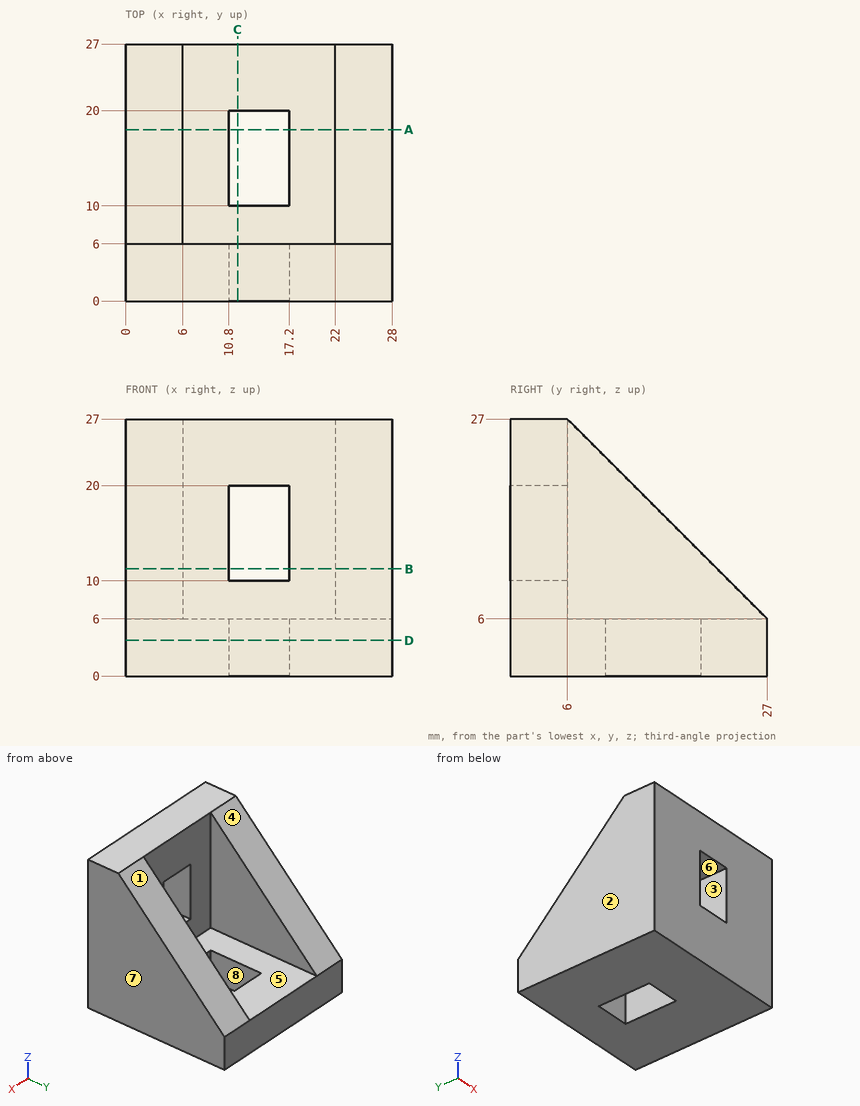
Design review of the part shown in the three views and the two pictorial views. Dimensions are in mm from the part's minimum x, y and z. A direction names the side the tool comes from. Round coordinates to 2 decimals unless told otherwise and drop trailing zeros. Write each loop counter-clockwise with the first axis right and the second up, starting at its lowest first coordinate (ties: lowest second). Pieces come first, ordered by that corner, then holes. Notation, with made-up numbers: (89.25, -20) - (122.25, -20) arc R33 ccw to (122.25, 8) - close; hole circle Ø5 at (-17, 0). An arc over 180 degrees is marked (long way). Write item = value, one per line. Start each with the question number.
1. Consider section D-D on z = 3.75. State the section outline as (x, y) points.
2. For pin 1 Ø3 at (y, z) = (15.5, 21.5) entering from +X; pin 2 Ø8 at (x, z) = (15.5, 17.5) entering from +Y; pin 3 Ø8 at (x, y) = (12.5, 13.5) entering from +Z, all flat-tipped, find the tip position at first contact; note any pin that passes through.
3. For the marked faces 4, 5, 6, 7 and 8, list the 3-axis set-ups (+Z, -Z, +X, -X, +Y, -Y) from which the entire face can be reached by the end or side of a thin tool; tool diameter is ignored.
4. Consider section B-B on z = 11.25. State the section outline as (x, y) points.
5. Consider section A-A on y = 18. State the section outline as (x, z) points, plus the area to 3 significant figures.
6. Wall thickness on L1, parallel to X at y = 1.25, z = 12; L2, parallel to X at y = 11.5, z = 8.25; L3, parallel to Y at x = 20, z = 25.5: over which ranges is each line inside the solid? List them lowest first.
7. Consider section C-C on x = 11.75. State the section outline as (y, z) points.
8. Draft analysis for pull direction X (two halves, no side actions). For the marked faces 1, 2 and 3, state which applies: released by +X, released by -X, zero draft, split by the parting line, or undercut.
Evaluation:
q1.outline = (0, 0) - (28, 0) - (28, 27) - (0, 27) - close; hole (10.8, 10) - (17.2, 10) - (17.2, 20) - (10.8, 20) - close
q2.pin_1 = through
q2.pin_2 = 6
q2.pin_3 = 6
q3.face_4 = +Z, +X, -X, +Y
q3.face_5 = +Z, +Y
q3.face_6 = +Y, -Y
q3.face_7 = +Z, -Z, +X, +Y, -Y
q3.face_8 = +Z, -Z
q4.outline = (0, 0) - (10.8, 0) - (10.8, 6) - (6, 6) - (6, 21.75) - (0, 21.75) - close; (17.2, 0) - (28, 0) - (28, 21.75) - (22, 21.75) - (22, 6) - (17.2, 6) - close
q5.outline = (0, 0) - (10.8, 0) - (10.8, 6) - (6, 6) - (6, 15) - (0, 15) - close; (17.2, 0) - (28, 0) - (28, 15) - (22, 15) - (22, 6) - (17.2, 6) - close
q5.area = 238 mm2
q6.L1 = 0 to 10.8, 17.2 to 28
q6.L2 = 0 to 6, 22 to 28
q6.L3 = 0 to 6
q7.outline = (0, 0) - (10, 0) - (10, 6) - (6, 6) - (6, 10) - (0, 10) - close; (0, 20) - (6, 20) - (6, 27) - (0, 27) - close; (20, 0) - (27, 0) - (27, 6) - (20, 6) - close
q8.face_1 = zero draft
q8.face_2 = released by -X
q8.face_3 = undercut
